Source: CAD feature listing. Evaluate the final solid. Frame: model axes, mm. Face numbers are marked on the shaded views. A direction names the side the tool comes from. Give positions to 0.01 mm unless a question says otherwise; leave off trailing zeros. Write each loop counter-clockwise with the first axis right and the second up, starting at its lowest first coordinate (ties: lowest second). Pieces come first, ordered by that corner, then holes. Notation, with made-up numbers: M 21.5,-26 L 50.5,-26 A16 cw 50.5,-1 Z; hole C 20,8 d10. An arc over 180 degrees is marked long. Return JSON: item names as keys, results as strings.
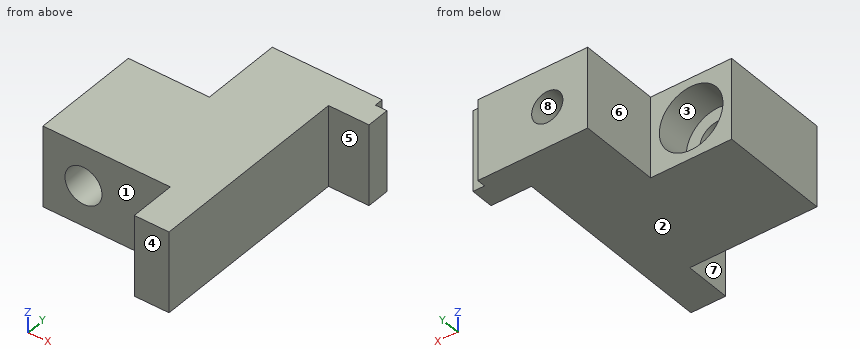
```python
from build123d import *

# Parameters (mm, degrees)
SALIENTE_EXTRUIR1_DEPTH = 7
CROQUIS4_R              = 1.35
CORTAR_EXTRUIR1_DEPTH   = 13.5
CROQUIS5_R              = 1.6
CORTAR_EXTRUIR2_DEPTH   = 13.9
CROQUIS6_R              = 2.75
CORTAR_EXTRUIR3_DEPTH   = 3


with BuildPart() as part:
    # Croquis1 → Saliente-Extruir1 (new body)
    with BuildSketch(Plane.XY):
        Polygon((0, 0), (4, 0), (4, -4), (7, -4), (7, 0), (7, 13.75), (10.5, 13.75), (10.5, 15.75), (9.5, 15.75), (9.5, 16.5), (7, 16.5), (0, 16.5), (0, 9.5), (-7, 9.5), (-7, 0), align=None)
    extrude(amount=SALIENTE_EXTRUIR1_DEPTH)

    # Croquis4 → Cortar-Extruir1 (cut)
    with BuildSketch(Plane(origin=(0, 16.5, 0), x_dir=(1, 0, 0), z_dir=(0, 1, 0))):
        with Locations(Location((3.5, -3.5, 0), (0, 0, 270))):
            Circle(CROQUIS4_R)
    extrude(amount=-CORTAR_EXTRUIR1_DEPTH, mode=Mode.SUBTRACT)

    # Croquis5 → Cortar-Extruir2 (cut)
    with BuildSketch(Plane(origin=(0, 9.5, 0), x_dir=(1, 0, 0), z_dir=(0, 1, 0))):
        with Locations(Location((-3.5, -3.5, 0), (0, 0, 180))):
            Circle(CROQUIS5_R)
    extrude(amount=-CORTAR_EXTRUIR2_DEPTH, mode=Mode.SUBTRACT)

    # Croquis6 → Cortar-Extruir3 (cut)
    with BuildSketch(Plane(origin=(0, 9.5, 0), x_dir=(1, 0, 0), z_dir=(0, 1, 0))):
        with Locations(Location((-3.5, -3.5, 0), (0, 0, 180))):
            Circle(CROQUIS6_R)
    extrude(amount=-CORTAR_EXTRUIR3_DEPTH, mode=Mode.SUBTRACT)


solid = part.part
```
1) Contact query for flat-ended pins moving along their axis: pin 1 Ø1.1 at (x, z) = (10, 5) entering from +Y; pin 2 Ø1.8 at (x, z) = (8.5, 3) entering from -Y; pin 3 Ø1.6 at (x, z) = (-4.5, 4.5) entering from +Y; pin 4 Ø2 at (y, z) = (-3, 3) entering from -X. Output: stop coordinate, or through.
Numbers:
{"pin 1": "stops at y = 16.5", "pin 2": "stops at y = 13.75", "pin 3": "stops at y = 6.5", "pin 4": "stops at x = 4"}
2) Cut plane D-D, the plane z = 0.5. Return the cut outline in (x, y).
Numbers:
{"outline": "M -7,0 L 4,0 L 4,-4 L 7,-4 L 7,13.75 L 10.5,13.75 L 10.5,15.75 L 9.5,15.75 L 9.5,16.5 L 0,16.5 L 0,9.5 L -7,9.5 Z"}
3) Cut plane C-C, the plane y = 9.25. Return the cut outline in (x, z), then the cut area to 3 significant figures.
Numbers:
{"outline": "M -7,0 L 7,0 L 7,7 L -7,7 Z; hole C -3.5,3.5 d5.5; hole C 3.5,3.5 d2.7", "area": "68.5 mm²"}
4) Cut plane A-A, the plane x = -3.5. Return the cut outline in (y, z), then the cut area to 3 significant figures.
Numbers:
{"outline": "M 0,0 L 9.5,0 L 9.5,0.75 L 6.5,0.75 L 6.5,1.9 L 0,1.9 Z; M 0,5.1 L 6.5,5.1 L 6.5,6.25 L 9.5,6.25 L 9.5,7 L 0,7 Z", "area": "29.2 mm²"}
5) Cut plane B-B, the plane z = 3.5. Return the cut outline in (x, y).
Numbers:
{"outline": "M -7,0 L -5.1,0 L -5.1,6.5 L -6.25,6.5 L -6.25,9.5 L -7,9.5 Z; M -1.9,0 L 4,0 L 4,-4 L 7,-4 L 7,13.75 L 10.5,13.75 L 10.5,15.75 L 9.5,15.75 L 9.5,16.5 L 4.85,16.5 L 4.85,3 L 2.15,3 L 2.15,16.5 L 0,16.5 L 0,9.5 L -0.75,9.5 L -0.75,6.5 L -1.9,6.5 Z"}
6) Line query: line 1 (X direction, y = 5, z = 4.5); line 2 (X direction, y = 10.75, z = 1.25); line 3 (Z direction, x = -3.5, y = 8.2). Output: solid intervals per line, ascending. Write a range as [from, to].
Numbers:
{"line 1": "x = [-7, -4.75], [-2.25, 2.59], [4.41, 7]", "line 2": "x = [0, 7]", "line 3": "z = [0, 0.75], [6.25, 7]"}
7) Draft query along Z for the marked faces 1, 2 and 3. Return one class per face: released by +Z, released by -Z, zero draft, split by the parting line, or undercut.
Numbers:
{"face 1": "zero draft", "face 2": "released by -Z", "face 3": "undercut"}
8) Set-up query: the marked faces 4, 5, 6, 7 and 8. Return all of +Z, -Z, +X, -X, +Y, -Y with unobstructed straight access to the full face (end or side cutting, diameter ignored); none if empty.
Numbers:
{"face 4": "+Z, -Z, +X, -X, -Y", "face 5": "+Z, -Z, +X, -Y", "face 6": "+Z, -Z, -X, +Y", "face 7": "+Z, -Z, -X, -Y", "face 8": "+Y"}
